Autodesk Inventor part; units mm, degrees
ref_plane "Work Plane1" through (0, 0, 5) normal (0, 0, 1) x (1, 0, 0)
ref_plane "YZ Plane" through (0, 0, 0) normal (1, 0, 0) x (0, 1, 0)
ref_plane "XZ Plane" through (0, 0, 0) normal (0, 1, 0) x (-1, 0, 0)
sketch "Sketch1" plane through (0, 0, 0) normal (0, 0, 1) x (1, 0, 0)
  line L0 (0, 0) -> (0, -15) construction
  line L1 (-5, 0) -> (-5, -15)
  line L2 (5, -15) -> (5, 0)
  arc A0 (5, 0) -> (-5, 0) centre (0, 0) ccw
  arc A1 (-5, -15) -> (5, -15) centre (0, -15) ccw
  line L3 (0, 0) -> (0, -15) construction
  line L4 (-10, 0) -> (-10, -15)
  line L5 (10, -15) -> (10, 0)
  arc A2 (10, 0) -> (-10, 0) centre (0, 0) ccw
  line L6 (0, -15) -> (0, -87) construction
  line L7 (5, -23.6603) -> (5, -82)
  line L8 (-5, -23.6603) -> (-5, -82)
  arc A3 (-10, -15) -> (-5, -23.6603) centre (0, -15) ccw
  arc A4 (5, -23.6603) -> (10, -15) centre (0, -15) ccw
  line L9 (-20, -82) -> (60, -82)
  line L10 (60, -82) -> (60, -87)
  line L11 (60, -87) -> (-20, -87)
  line L12 (-20, -87) -> (-20, -82)
  circle A5 centre (0, 0) radius 5
  circle A6 centre (0, 0) radius 10
  line L13 (-5, -23.6603) -> (-5, 8.6603)
  line L14 (5, -23.6603) -> (5, 8.6603)
  point P0 (0, -7.5)
  point P1 (0, -7.5)
  point P2 (5, 0)
  point P3 (5, -8.6603)
  point P4 (-5, -8.6603)
  dimension "d0" = 15
  dimension "d1" = 5
  dimension "d2" = 10
  dimension "d3" = 72
  dimension "d4" = 5
  dimension "d5" = 5
  dimension "d7" = 80
  dimension "d8" = 5
  dimension "d24" = 15
extrude "Extrusion1" add sketch "Sketch1" along normal blind 10 contours A5 L2 A6 L1 | L13 A2 L14 A0 | L1 A6 A2 L13 | A6 L2 A1 L1 | L14 A2 A6 L2 | A1 L14 L7 L9 L8 L13 | L9 L10 L11 L12
sketch "Sketch2" plane through (0, 0, 0) normal (0, 0, -1) x (-1, 0, 0)
  arc A0 (-5, -15) -> (5, -15) centre (0, -15) ccw
  line L0 (0, 0) -> (0, -15) construction
  line L1 (-10, 0) -> (-10, -15)
  line L2 (10, -15) -> (10, 0)
  arc A1 (10, 0) -> (-10, 0) centre (0, 0) ccw
  arc A2 (-10, -15) -> (10, -15) centre (0, -15) ccw
  line L3 (0, 0) -> (0, -15) construction
  line L4 (-5, 0) -> (-5, -15)
  line L5 (5, -15) -> (5, 0)
  arc A3 (5, 0) -> (-5, 0) centre (0, 0) ccw
  arc A4 (-5, -15) -> (5, -15) centre (0, -15) ccw
  circle A5 centre (0, 0) radius 10
  circle A6 centre (0, 0) radius 5
  point P0 (0, -7.5)
  point P1 (0, -7.5)
  point P2 (-5, -15)
  dimension "d11" = 10
  dimension "d12" = 5
extrude "Extrusion2" add sketch "Sketch2" along normal blind 8 contours A5 A1 L5 A3 L4 | L4 A6 L5 A5
sketch "Sketch3" plane through (0, 0, 10) normal (0, 0, 1) x (1, 0, 0)
  line L0 (-20, -82) -> (-20, -87)
  line L1 (-20, -87) -> (60, -87)
  line L2 (-20, -82) -> (60, -82)
  line L3 (60, -82) -> (60, -87)
  line L4 (60, -87) -> (-20, -87)
  line L5 (-20, -87) -> (-20, -82)
  point P0 (0, 0)
  dimension "d23" = 80
extrude "Extrusion3" add sketch "Sketch3" along normal blind 3
ref_plane "Work Plane1" through (0, 0, 5) normal (0, 0, 1) x (1, 0, 0)
sketch "Sketch4" plane through (0, 0, 5) normal (0, 0, 1) x (1, 0, 0)
  arc A0 (-20, -82) -> (-5, -67) centre (-20, -67) ccw
  line L0 (-5, -23.6603) -> (-5, -82)
  line L1 (60, -82) -> (-20, -82)
  line L2 (-5, -67) -> (-20, -67) construction
  line L3 (-20, -67) -> (-20, -82) construction
  line L4 (-20, -82) -> (-5, -82)
  line L5 (-5, -82) -> (-5, -67)
  arc A1 (5, -63) -> (16.8392, -77.6632) centre (20, -63) ccw
  line L6 (5, -82) -> (5, -23.6603)
  line L7 (16.8392, -77.6632) -> (36.9579, -82)
  line L8 (5, -82) -> (5, -63)
  point P0 (0, 0)
  point P1 (-20, -82)
  dimension "d17" = 15
  dimension "d18" = 30
  dimension "d20" = 19
extrude "Extrusion4" add sketch "Sketch4" along normal mid plane 4
equation "\"d9\" = d2"
properties part number "Stand" material "Steel, Mild"
Work out the finished part from the listing and answer in its coordinate system (mm). A direction names the side the tool comes from. Coordinates: 2 decimals unless noted, no trailing zeros. Write each loop counter-clockwise with the first axis right and the second up, starting at its lowest first coordinate (ties: lowest second). Pieces come first, ordered by that corner, then holes. Notation, with made-up numbers: M 18.25,67.25 L 62.25,67.25 A22 cw 62.25,90.25 Z; hole C -1.75,30.5 d9. An arc over 180 degrees is marked long. Write item = value, one per line.
1. Flat-ended cylindrical pins translate along their axes: pin 1 (2 mm diameter, centred on x = -1, y = -35, fed in from +Z); pin 2 (1 mm diameter, centred on x = 21.5, z = 6.5, fed in from +Y); pin 3 (1.5 mm diameter, centred on x = -15, z = 2, fed in from +Y). Find the tip coordinate at first contact, or state that the pin passes through.
Solution:
pin_1 = 10
pin_2 = -78.56
pin_3 = -82
2. The part is cut by section B-B (z = 4.75). Determine the outline of the cut face in (x, y).
Solution:
outline = M -20,-87 L 60,-87 L 60,-82 L 36.96,-82 L 16.84,-77.66 A15 cw 5,-63 L 5,-8.66 A10 ccw long -5,-8.66 L -5,-67 A15 cw -20,-82 Z; hole C 0,0 d10
3. Straight lines are drawn through the part: line 1 (X direction, y = 0, z = -3.75); line 2 (Y direction, x = 0, z = 6.75); line 3 (X direction, y = -18.5, z = 4.5). For each, find the intervals that lie inside material, in ascending order. Write a range as from..to.
Solution:
line_1 = -10..-5, 5..10
line_2 = -87..-5, 5..10
line_3 = -5..5
4. For faces 1 (the face through (0, -35, 10)), 2 (the face through (8.419, -72.534, 4.972)), 3 (the face through (-8, -79, 7)), determine the directions among +Z, -Z, +X, -X, +Y, -Y from which every point of the face is accessible in a straight line to the end or side of a thin tool.
Solution:
face_1 = +Z, +X, -X, +Y
face_2 = +Z, -Z, +X
face_3 = +Z, -X
5. The part is cut by section A-A (x = 8). Determine the outline of the cut face in (y, z).
Solution:
outline = M -87,0 L -82,0 L -82,3 L -72,3 L -72,7 L -82,7 L -82,13 L -87,13 Z; M -6,-8 L 6,-8 L 6,10 L -6,10 Z
6. The part is cut by section C-C (y = 0). Determine the outline of the cut face in (x, z).
Solution:
outline = M -10,-8 L -5,-8 L -5,10 L -10,10 Z; M 5,-8 L 10,-8 L 10,10 L 5,10 Z
7. The part is cut by section D-D (x = 0). Determine the outline of the cut face in (y, z).
Solution:
outline = M -87,0 L -10,0 L -10,-8 L -5,-8 L -5,10 L -82,10 L -82,13 L -87,13 Z; M 5,-8 L 10,-8 L 10,10 L 5,10 Z
8. Determine the mould class of faces 4 (the face through (5, -46, 5)), 5 (the face through (19, -87, 6)), 6 (the face through (26.76, -79.8, 4.97)), 7 (the face through (2, -62, 0)) for opening direction Y: released by +Y, released by -Y, zero draft, split by the parting line, or undercut.
Solution:
face_4 = undercut
face_5 = released by -Y
face_6 = released by +Y
face_7 = zero draft
